Geometry check sheet. Reference: drawing and pictorial views, mm from the part's lowest x, y, z. Give positions to 0.01 mm unless a question says otherwise; leave off trailing zeros. Loops run counter-clockwise (first coordinate to the right, second up) from the corner with the lowest first, then second, coordinate; pieces in that order, holes last. Notation, with made-up numbers: (-23.5, 89.25) -> (12.5, 89.25) arc R20 cw to (12.5, 120.25) -> close; hole circle Ø4 at (14.5, 54). An arc over 180 degrees is marked (long way). Write each question's results on one line, items separated by ' | '. Start each with the question number.
1. Cross-section at A-A on z = 33. Record the boundary of the cut face in (x, y).
2. Mould release check, pull along Z, two halves, no side actions. Record for the marked faces 1, 2, 3 and 4: +Z half, -Z half, draft (parallel to the pull), parting line (faces both ways), or undercut.
3. Cross-section at C-C on x = 4. Record the boundary of the cut face in (y, z).
4. Cross-section at B-B on y = 56.5. Count the separate pieces of the cut face and the enclosed holes in it.
5. Gauge pin test, flat ends, axial feed: pin 1 Ø2 at (x, z) = (23.5, 21.5) entering from +Y; pin 2 Ø6 at (x, y) = (15, 23) entering from +Z (1 decimal); pin 3 Ø5 at (x, y) = (33.5, 17.5) entering from +Z; pin 4 Ø2 at (x, z) = (56.63, 53.47) entering from +Y. Record the tip position at first contact, or that the pin passes through.
6. Material ranges on L1, parallel to Z at x = 33, y = 17 (1 decimal); L2, parallel to Z at x = 32.5, y = 10 (1 decimal); L3, parallel to Y at x = 20, z = 43, recorded low to high. Write a range as from..to.
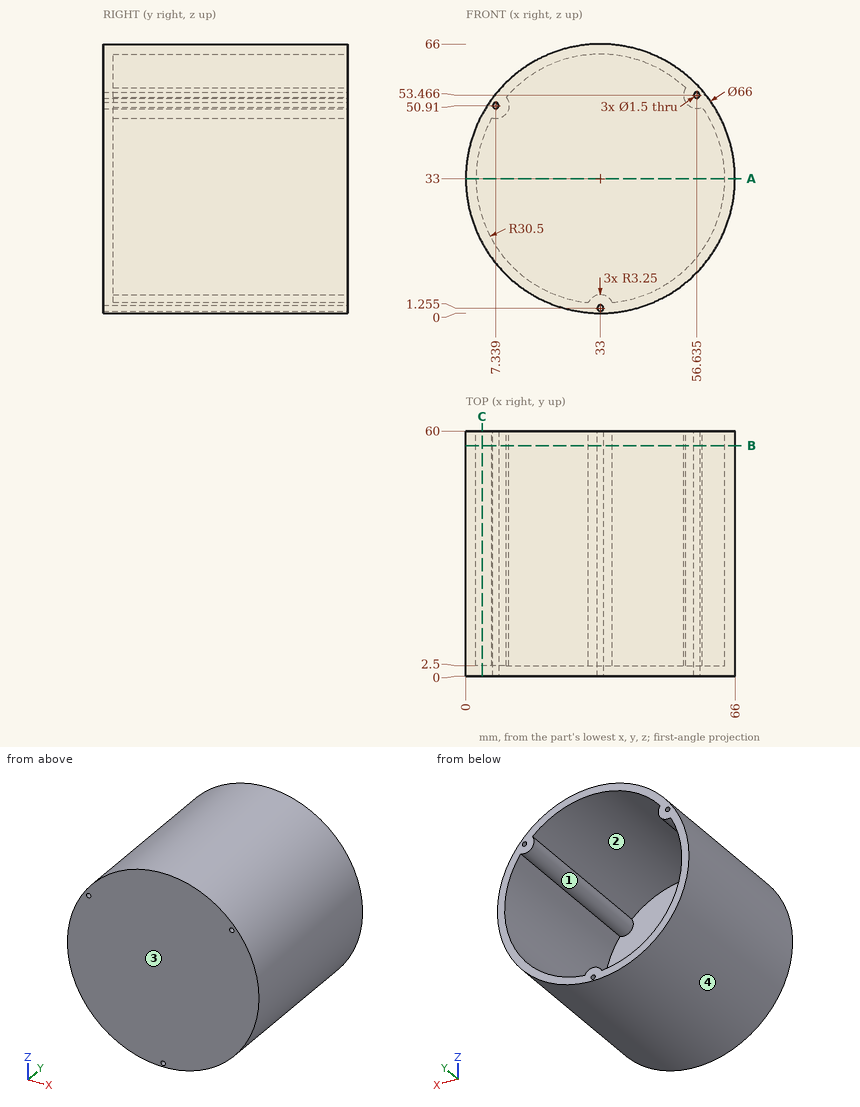
Geometry says:
1) outline: (0, 0) -> (66, 0) -> (66, 60) -> (63.5, 60) -> (63.5, 2.5) -> (2.5, 2.5) -> (2.5, 60) -> (0, 60) -> close
2) face 1: undercut | face 2: undercut | face 3: draft | face 4: parting line
3) outline: (0, 17.25) -> (60, 17.25) -> (60, 23.55) -> (2.5, 23.55) -> (2.5, 42.45) -> (60, 42.45) -> (60, 48.75) -> (0, 48.75) -> close
4) separate pieces: 1 | enclosed holes: 4
5) pin 1: y = 2.5 | pin 2: z = 62.4 | pin 3: z = 66 | pin 4: y = 60
6) L1: 0..0.5, 2..4.5, 63.5..66 | L2: 0..0.7, 1.8..4.5, 63.5..66 | L3: 0..2.5
